Can you work these out from the model? Positions are in its coordinate system, mm. A direction names the side the tool comes from. Give positions to 0.01 mm unless a question says otherwise; leave off trailing zeros. Order: outer loops, then holes, each group sorted by start corner. A loop starts at its lowest first (then second) coordinate and runs counter-clockwise, first axis right, second up. Notation, with made-up numbers: (72.25, -12) - (120.25, -12) arc R11 ccw to (120.25, -5) - close; hole circle Ø11 at (82.5, -1.5). An arc over 180 degrees is marked (long way). Return JSON: item names as keys, results as strings.
```python
from build123d import *

# Parameters (mm, degrees)
SKETCH1_R           = 10
BOSS_EXTRUDE1_DEPTH = 61
SKETCH2_W           = 39.5
SKETCH2_H           = 2.5
SKETCH3_W           = 25
SKETCH3_H           = 1.5
SKETCH4_W           = 1.1
SKETCH4_H           = 0.6
SKETCH5_W           = 1.3
SKETCH5_H           = 0.75


with BuildPart() as part:
    # Sketch1 → Boss-Extrude1 (new, symmetric)
    with BuildSketch(Plane.XY):
        with Locations(Location((0, 0, 0), (0, 0, 180))):
            Circle(SKETCH1_R)
    extrude(amount=BOSS_EXTRUDE1_DEPTH, both=True)

    # Sketch2 → Cut-Revolve1 (revolve, cut)
    with BuildSketch(Plane(origin=(0, 0, 0), x_dir=(0, 0, -1), z_dir=(1, 0, 0)), mode=Mode.PRIVATE) as cut_revolve1_sk:
        with Locations((41.25, 8.75)):
            Rectangle(SKETCH2_W, SKETCH2_H)
    cut_revolve1 = revolve(cut_revolve1_sk.sketch.rotate(Axis((0, 0, -67.1), (0, 0, 1)), 90), axis=Axis((0, 0, -67.1), (0, 0, 1)), mode=Mode.SUBTRACT)

    # Mirror1: Cut-Revolve1 across plane
    add(cut_revolve1.mirror(Plane.XY), mode=Mode.SUBTRACT)

    # Sketch3 → Cut-Revolve2 (revolve, cut)
    with BuildSketch(Plane(origin=(0, 0, 0), x_dir=(0, 0, -1), z_dir=(1, 0, 0)), mode=Mode.PRIVATE) as cut_revolve2_sk:
        with Locations((48.5, 6.75)):
            Rectangle(SKETCH3_W, SKETCH3_H)
    cut_revolve2 = revolve(cut_revolve2_sk.sketch.rotate(Axis((0, 0, -67.1), (0, 0, 1)), 90), axis=Axis((0, 0, -67.1), (0, 0, 1)), mode=Mode.SUBTRACT)

    # Mirror2: Cut-Revolve2 across plane
    add(cut_revolve2.mirror(Plane.XY), mode=Mode.SUBTRACT)

    # Sketch4 → Cut-Revolve3 (revolve, cut)
    with BuildSketch(Plane(origin=(0, 0, 0), x_dir=(0, 0, -1), z_dir=(1, 0, 0)), mode=Mode.PRIVATE) as cut_revolve3_sk:
        with Locations((30.95, 7.2)):
            Rectangle(SKETCH4_W, SKETCH4_H)
    cut_revolve3 = revolve(cut_revolve3_sk.sketch.rotate(Axis((0, 0, -67.1), (0, 0, 1)), 90), axis=Axis((0, 0, -67.1), (0, 0, 1)), mode=Mode.SUBTRACT)

    # Mirror3: Cut-Revolve3 across plane
    add(cut_revolve3.mirror(Plane.XY), mode=Mode.SUBTRACT)

    # Sketch5 → Cut-Revolve4 (revolve, cut)
    with BuildSketch(Plane(origin=(0, 0, 0), x_dir=(0, 0, -1), z_dir=(1, 0, 0)), mode=Mode.PRIVATE) as cut_revolve4_sk:
        with Locations((10.55, 9.625)):
            Rectangle(SKETCH5_W, SKETCH5_H)
    cut_revolve4 = revolve(cut_revolve4_sk.sketch.rotate(Axis((0, 0, -67.1), (0, 0, 1)), 90), axis=Axis((0, 0, -67.1), (0, 0, 1)), mode=Mode.SUBTRACT)

    # Mirror4: Cut-Revolve4 across plane
    add(cut_revolve4.mirror(Plane.XY), mode=Mode.SUBTRACT)


solid = part.part
```
1. On a 3-axis mill with a long thin cutter (end or side, diameter ignored), from which of +Z, -Z, +X, -X, +Y, -Y can I reach the whole of each face in a straight line? I mean faces 4 (the face through (-4.032, -6.324, 26.012)), 5 (the face through (-4.268, 8.206, 10.559)), 6 (the face through (4, -7, -21.5)). Say none if no direction works.
Checks:
{"face 4": "+Z", "face 5": "none", "face 6": "-Z"}
2. Thinking about a two-plate mould opening in Z: for faces 1 (the face through (2, -6, 36)), 2 (the face through (2, -6, -36)), 3 (the face through (7, 2, 30.4)), which applies, +Z half, -Z half, draft (parallel to the pull), parting line (faces both ways), or undercut?
Checks:
{"face 1": "+Z half", "face 2": "-Z half", "face 3": "undercut"}
3. For pin 1 Ø8 at (x, z) = (-5.5, -20.5) entering from -Y; pin 2 Ø1 at (x, z) = (4.5, -15.5) entering from +Y; pin 3 Ø3 at (y, z) = (6.5, -13.5) entering from -X, each with a flat end and sliding along its axis, tell me the tip position at first contact or that it passes through.
Checks:
{"pin 1": "y = -9.89", "pin 2": "y = 9.17", "pin 3": "x = -8.66"}
4. If I drill on L1, parallel to Z at x = 8.5, y = -3.5; L2, parallel to Y at x = 0.25, z = -3; L3, parallel to X at y = -1.5, z = -14, over which ranges is the centre line in solid material (lowest first)? Write a range as [from, to].
Checks:
{"L1": "[-21.5, 21.5]", "L2": "[-10, 10]", "L3": "[-9.89, 9.89]"}
5. Suppose I cut it at A-A (z = 40). List the corners of the cut face in (x, y) for me.
Checks:
{"outline": "circle Ø12 at (0, 0)"}
6. Suppose I cut it at B-B (z = 2.5). List the corners of the cut face in (x, y) for me, plus the area to 3 significant figures.
Checks:
{"outline": "circle Ø20 at (0, 0)", "area": "314 mm^2"}
